Can you work these out from the model? Positions are in its coordinate system, mm. A direction names the side the tool comes from. Round coordinates to 2 decimals unless told otherwise and drop trailing zeros. Loops run counter-clockwise (first coordinate to the right, second up) from the corner with the lowest first, then second, coordinate; pieces in that order, holes last.
from build123d import *

# Parameters (mm, degrees)
SKETCH1_R           = 254
BOSS_EXTRUDE1_DEPTH = 508
BOSS_EXTRUDE2_DEPTH = 1016


with BuildPart() as part:
    # Sketch1 → Boss-Extrude1 (new body)
    with BuildSketch(Plane.XY):
        with BuildLine():
            Line((0, 0), (1370.792512001, 0))
            Line((1370.792512001, 0), (1370.792512001, 254))
            ThreePointArc((1370.792512001, 254), (1296.397634423, 433.605122421), (1116.792512001, 508))
            Line((1116.792512001, 508), (1016, 508))
            ThreePointArc((1016, 508), (508, 1016), (0, 508))
            Line((0, 508), (0, 0))
        make_face()
        with Locations((508, 508)):
            Circle(SKETCH1_R, mode=Mode.SUBTRACT)
    extrude(amount=BOSS_EXTRUDE1_DEPTH)

    # Sketch1<4> → Boss-Extrude2 (add)
    with BuildSketch(Plane.XY):
        Polygon((0, 254), (0, 0), (1370.792512001, 0), (1370.792512001, 254), (508, 254), align=None)
    extrude(amount=BOSS_EXTRUDE2_DEPTH)


solid = part.part
(1) If we section it at A-A, the plane y = 491: List the corners of the cut face in (x, z) for me, then the cut area to 3 significant figures.
Worked answers:
outline: (0, 0) - (254.57, 0) - (254.57, 508) - (0, 508) - close; (761.43, 0) - (1208.15, 0) - (1208.15, 508) - (761.43, 508) - close
area: 356,000 mm2
(2) If we section it at B-B, the plane z = 110: List the corners of the cut face in (x, y) for me, then the cut area to 3 significant figures.
Worked answers:
outline: (0, 0) - (1370.79, 0) - (1370.79, 254) arc R254 ccw to (1116.79, 508) - (1016, 508) arc R508 ccw to (0, 508) - close; hole circle Ø508 at (508, 508)
area: 885,000 mm2
(3) For faces 5 (the flat face through (676, 289, 0)), 6 (the flat face through (1067, 508, 250)), 7 (the flat face through (676, 725, 508)), which set-ups out of +Z, -Z, +X, -X, +Y, -Y let a thin tool reach every point of the face, with its end or its side?
Worked answers:
face 5: -Z, +X, -X, +Y, -Y
face 6: +Z, -Z, +X, +Y
face 7: +Z, +X, -X, +Y
(4) If we section it at D-D, the plane z = 899: List the corners of the cut face in (x, y) for me.
Worked answers:
outline: (0, 0) - (1370.79, 0) - (1370.79, 254) - (0, 254) - close
(5) If we mould it in two halves opening along X, with no side actions, what happens to faces 1 (the cylindrical face through (1298.36, 431.62, 250.44)), 2 (the cylindrical face through (254.246, 519.168, 250.444)), 3 (the flat face through (695, 254, 758)), 4 (the cylindrical face through (519.171, 1015.877, 250.444))? For each: released by +X, released by -X, zero draft, split by the parting line, or undercut.
Worked answers:
face 1: released by +X
face 2: undercut
face 3: zero draft
face 4: split by the parting line
(6) If we section it at C-C, the plane x = 588: List the corners of the cut face in (y, z) for me, then the cut area to 3 significant figures.
Worked answers:
outline: (0, 0) - (266.93, 0) - (266.93, 508) - (254, 508) - (254, 1016) - (0, 1016) - close; (749.07, 0) - (1009.66, 0) - (1009.66, 508) - (749.07, 508) - close
area: 397,000 mm2
(7) If I drill on line 1 (Y direction, x = 508, z = 373); line 2 (Z direction, x = 1298, y = 393); line 3 (Y direction, x = 794.5, z = 685), over which ranges is the centre line in solid material (lowest first)?
Worked answers:
line 1: y = 0 to 254, 762 to 1016
line 2: z = 0 to 508
line 3: y = 0 to 254
(8) Will these pins go through, and if not, where does the flat tip stop? P1, Ø5, axis at x = 464.5, y = 812, coming from the -Z side; P2, Ø6, axis at y = 315, z = 216, coming from the +X side; P3, Ø3, axis at x = 659.5, z = 524, coming from the +Y side; P4, Ø1, axis at x = 313, z = 368, coming from the +Y side.
Worked answers:
P1: stops at z = 0
P2: stops at x = 1364.08
P3: stops at y = 254
P4: stops at y = 977.29
